```python
from build123d import *

# Parameters (mm, degrees)
SKETCH1_R           = 15
BOSS_EXTRUDE3_DEPTH = 10
BOSS_EXTRUDE4_DEPTH = 10
SKETCH3_R           = 10
CUT_EXTRUDE1_DEPTH  = 1903.755203621


with BuildPart() as part:
    # Sketch1 → Boss-Extrude3 (new body)
    with BuildSketch(Plane.XY):
        with Locations((6.605137187, -1887.466420258)):
            Circle(SKETCH1_R)
        with BuildLine():
            Line((31.605137187, -1638.974115082), (-18.394862813, -1638.974115082))
            Line((-18.394862813, -1638.974115082), (-18.394862813, -1688.974115082))
            Line((-18.394862813, -1688.974115082), (-8.375934863, -1888.219733093))
            ThreePointArc((-8.375934863, -1888.219733093), (6.228361891, -1872.471152992), (21.605137187, -1887.466420258))
            ThreePointArc((21.605137187, -1887.466420258), (21.600404453, -1887.843195554), (21.586209238, -1888.219733093))
            Line((21.586209238, -1888.219733093), (31.605137187, -1688.974115082))
            Line((31.605137187, -1688.974115082), (31.605137187, -1638.974115082))
        make_face()
    extrude(amount=BOSS_EXTRUDE3_DEPTH)

    # Sketch2 → Boss-Extrude4 (add)
    with BuildSketch(Plane(origin=(0, 0, 0), x_dir=(-1, 0, 0), z_dir=(0, 0, -1))):
        with BuildLine():
            Line((-31.605137187, -1638.974115082), (18.394862813, -1638.974115082))
            ThreePointArc((18.394862813, -1638.974115082), (-6.605137187, -1613.974115082), (-31.605137187, -1638.974115082))
        make_face()
    extrude(amount=-BOSS_EXTRUDE4_DEPTH)

    # Sketch3 → Cut-Extrude1 (cut, through all)
    with BuildSketch(Plane(origin=(0, 0, 0), x_dir=(-1, 0, 0), z_dir=(0, 0, -1))):
        with Locations((-6.605137187, -1668.974115082)):
            Circle(SKETCH3_R)
    extrude(amount=-CUT_EXTRUDE1_DEPTH, mode=Mode.SUBTRACT)


solid = part.part
```
Input: part model. Units: mm. Frame: model coordinates. Give positions to 0.01 mm unless a question says otherwise; leave off trailing zeros. Order: outer loops, then holes, each group sorted by start corner. A loop starts at its lowest first (then second) coordinate and runs counter-clockwise, first axis right, second up. Notation, with made-up numbers: M 68,82 L 73,82 A23 cw 73,91 Z; hole C 50,9 d8. An arc over 180 degrees is marked long. Return JSON: item names as keys, results as strings.
1) Contact query for flat-ended pins moving along their axis: pin 1 (4 mm diameter, centred on x = 15.5, z = 6.5, fed in from -Y); pin 2 (4 mm diameter, centred on x = 16, z = 6.5, fed in from +Y); pin 3 (2 mm diameter, centred on y = -1719.5, z = 6.5, fed in from -X). Output: stop coordinate, or through.
Taken from the geometry:
{"pin 1": "stops at y = -1900.79", "pin 2": "stops at y = -1615.09", "pin 3": "stops at x = -16.91"}
2) Section query D-D on x = 25.5. Output: boundary loops of the cut face in (y, z), and give its area (3 significant figures).
Taken from the geometry:
{"outline": "M -1810.39,0 L -1622.6,0 L -1622.6,10 L -1810.39,10 Z", "area": "1,880 mm2"}
3) Section query A-A on y = -1664.5. Output: boundary loops of the cut face in (x, z).
Taken from the geometry:
{"outline": "M -18.39,0 L -2.34,0 L -2.34,10 L -18.39,10 Z; M 15.55,0 L 31.61,0 L 31.61,10 L 15.55,10 Z"}
4) Section query C-C on z = 7. Output: boundary loops of the cut face in (x, y), and give its area (3 significant figures).
Taken from the geometry:
{"outline": "M -18.39,-1688.97 L -8.38,-1888.22 A15 ccw 21.59,-1888.22 L 31.61,-1688.97 L 31.61,-1638.97 A25 ccw -18.39,-1638.97 Z; hole C 6.61,-1668.97 d20", "area": "11,500 mm2"}
5) Mould query, pull axis Y, two halves, no side actions, for faces 1 (the face through (7.91, -1659.06, 4.93)), 2 (the face through (-13.456, -1787.202, 4.93)), 3 (the face through (7, -1756, 0)). Classes: released by +Y, released by -Y, zero draft, split by the parting line, or undercut.
Taken from the geometry:
{"face 1": "undercut", "face 2": "released by -Y", "face 3": "zero draft"}
6) Section query B-B on x = 13. Output: boundary loops of the cut face in (y, z).
Taken from the geometry:
{"outline": "M -1901.03,0 L -1676.66,0 L -1676.66,10 L -1901.03,10 Z; M -1661.29,0 L -1614.81,0 L -1614.81,10 L -1661.29,10 Z"}
7) Line query: L1, parallel to Y at x = 0, z = 6.25; L2, parallel to Y at x = 12.5, z = 4.5; L3, parallel to X at y = -1743.5, z = 5.5. Output: solid intervals per line, ascending. Write a range as [from, to].
Taken from the geometry:
{"L1": "y = [-1900.93, -1676.48], [-1661.47, -1614.86]", "L2": "y = [-1901.26, -1677.05], [-1660.9, -1614.68]", "L3": "x = [-15.65, 28.86]"}
